Autodesk Inventor part; units mm, degrees
ref_plane "YZ Plane" through (0, 0, 0) normal (1, 0, 0) x (0, 1, 0)
ref_plane "XZ Plane" through (0, 0, 0) normal (0, 1, 0) x (-1, 0, 0)
ref_plane "XY Plane" through (0, 0, 0) normal (0, 0, 1) x (1, 0, 0)
sketch "Sketch1" plane through (0, 0, 0) normal (0, 1, 0) x (-1, 0, 0)
  line L0 (0, 0) -> (-18.5, 0)
  line L1 (-18.5, 0) -> (-18.5, -42.5)
  line L2 (-18.5, -42.5) -> (0, -42.5)
  line L3 (0, -42.5) -> (0, 0)
  dimension "d0" = 18.5
  dimension "d1" = 42.5
extrude "Extrusion1" add sketch "Sketch1" along normal blind 4
sketch "Sketch2" plane through (0, 0, 0) normal (0, -1, 0) x (1, 0, 0)
  line L0 (0, -42.5) -> (0, 0)
  line L1 (18.5, 0) -> (18.5, -42.5)
  line L2 (0, 0) -> (18.5, 0)
  line L3 (18.5, 0) -> (18.5, -3)
  line L4 (18.5, -3) -> (0, -3)
  line L5 (0, -3) -> (0, 0)
  dimension "d4" = 3
extrude "Extrusion2" add sketch "Sketch2" along normal blind 18.5
sketch "Sketch3" plane through (0, 4, 0) normal (0, 1, 0) x (1, 0, 0)
  line L0 (1.2509, 3.5794) -> (17.7774, 3.5794) construction
  line L1 (17.7774, 3.5794) -> (17.7774, 0.9324) construction
  line L2 (17.7774, 0.9324) -> (1.2509, 0.9324) construction
  line L3 (1.2509, 0.9324) -> (1.2509, 3.5794) construction
  line L4 (7.0482, 14.2862) -> (7.0482, 39.4285) construction
  line L5 (7.0482, 39.4285) -> (10.2049, 39.4285) construction
  line L6 (10.2049, 39.4285) -> (10.2049, 14.2862) construction
  line L7 (10.2049, 14.2862) -> (7.0482, 14.2862) construction
  point P0 (0, 0)
  dimension "d2" = 4
  dimension "d3" = 0
properties part number "controller_reveiver"
Verification items for the finished model (mm, model axes). A direction names the side the tool comes from. Give positions to 0.01 mm unless a question says otherwise; leave off trailing zeros. Loops run counter-clockwise (first coordinate to the right, second up) from the corner with the lowest first, then second, coordinate; pieces in that order, holes last. Notation, with made-up numbers: (40.5, 30.25) - (46.5, 30.25) arc R22 cw to (46.5, 49.25) - close; hole circle Ø2 at (3, 62). An arc over 180 degrees is marked (long way). Write each question's results on one line, items separated by ' | '.
1) Depth check by flat-ended pin: P1, Ø10, axis at x = 12, y = -8.5, coming from the -Z side; P2, Ø3, axis at y = -2, z = -11, coming from the -X side; P3, Ø1.5, axis at x = 5.5, z = -33, coming from the -Y side. Enter the tip coordinate at first touch or a pass-through.
Solution:
P1: z = -3 | P2: through | P3: y = 0
2) Tool access check on faces 1 (the flat face through (9, -9, -3)), 2 (the flat face through (9, -18.5, -1)). Record the directions out of +Z, -Z, +X, -X, +Y, -Y that give a thin tool (end or side, any length) a straight path to the whole face; none if there is none.
Solution:
face 1: -Z, +X, -X, -Y | face 2: +Z, -Z, +X, -X, -Y
3) Sectioned sample at C-C on y = -6.5. Record the boundary of the cut face in (x, z), plus the area to 3 significant figures.
Solution:
outline: (0, -3) - (18.5, -3) - (18.5, 0) - (0, 0) - close | area: 55.5 mm2
4) Sectioned sample at A-A on z = -15. Record the boundary of the cut face in (x, y), plus the area to 3 significant figures.
Solution:
outline: (0, 0) - (18.5, 0) - (18.5, 4) - (0, 4) - close | area: 74.0 mm2
5) Material ranges on L1, parallel to Z at x = 4.25, y = -10.75; L2, parallel to Y at x = 15, z = -9, recorded low to high. Write a range as from..to.
Solution:
L1: -3..0 | L2: 0..4
6) Sectioned sample at B-B on x = 11.75. Record the boundary of the cut face in (y, z), plus the area to 4 significant figures.
Solution:
outline: (-18.5, -3) - (0, -3) - (0, -42.5) - (4, -42.5) - (4, 0) - (-18.5, 0) - close | area: 225.5 mm2
